Input: dimensioned drawing with shaded views. Units: mm. Origin: part minimum x, y, z. A direction names the side the tool comes from. Give positions to 0.01 mm unless a question says otherwise; leave off trailing zeros. Order: outer loops, then holes, each group sorted by start corner. A loop starts at its lowest first (then second) coordinate and runs counter-clockwise, first axis right, second up. Notation, with made-up numbers: M 73.5,12 L 114.5,12 A18 cw 114.5,32 Z; hole C 34,-23 d8. An arc over 180 degrees is marked long. Answer in a Markdown table with one row per item. Add a question column.
(1) Section query C-C, the plane z = 1.75. Return loops of the section in (x, y), plus the area to 3 significant figures.
(2) Section query A-A, the plane x = 8. Return loops of the section in (y, z).
(3) Material intervals for line 1 along Y through (x, z) = (8, 3.5); line 2 along Z through (x, y) = (2.25, 5.75); line 3 along X through (y, z) = (9.25, 5.75), sorted ascending.
(4) Mould query, pull axis Y, two halves, no side actions, for the marked faces 3, 4 and 5. Classes: pulls with the +Y half, pulls with the -Y half, needs draft (parallel to the pull), parting line crosses it, or undercut.
(5) Section query D-D, the plane z = 7.75. Return loops of the section in (x, y), plus the area to 3 significant figures.
(6) Set-up query: the marked faces 1 and 2. Return all of +Z, -Z, +X, -X, +Y, -Y with unobstructed straight access to the full face (end or side cutting, diameter ignored); none if empty.
(7) Pin query (flat end, axial travel): P1, Ø1.5, axis at x = 10.5, z = 2.5, coming from the +Y side; P2, Ø2, axis at y = 10.5, z = 2.5, coming from the -X side; P3, Ø2, axis at y = 9, z = 3.5, coming from the -X side. Return the tip coordinate at first contact, or that it passes through.
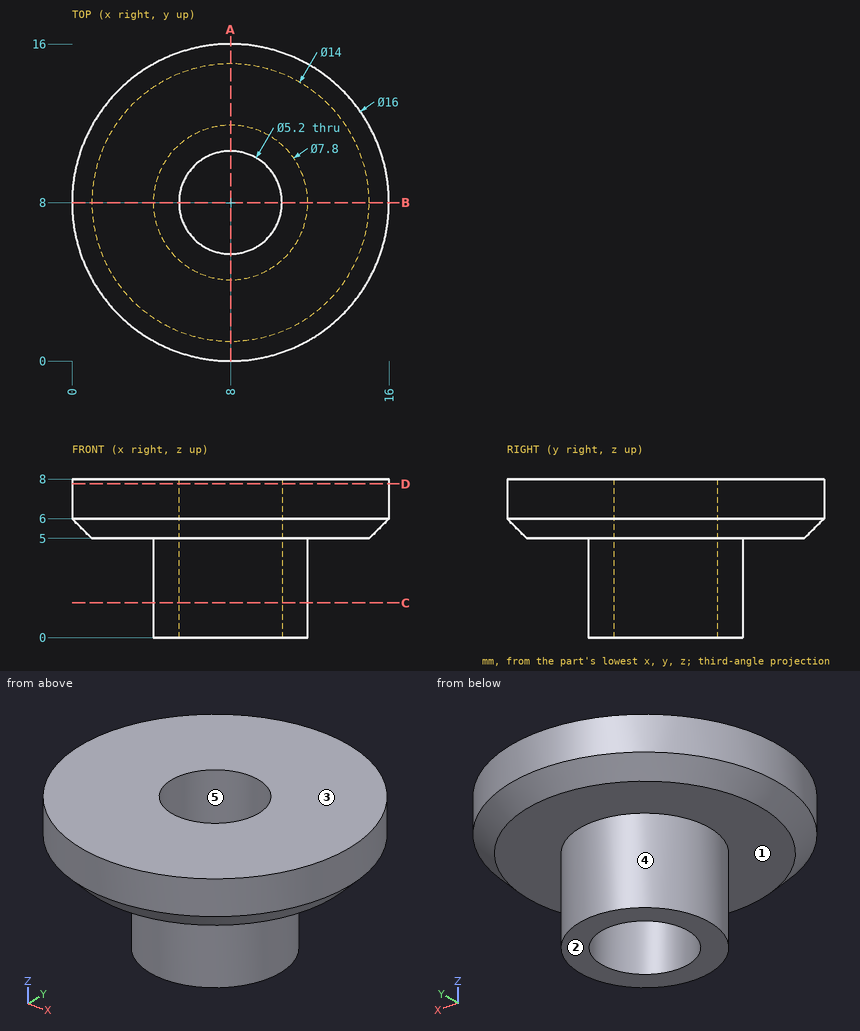
Values follow:
| question | item | result |
|---|---|---|
| 1 | outline | C 8,8 d7.8; hole C 8,8 d5.2 |
| 1 | area | 26.5 mm² |
| 2 | outline | M 0,6 L 1,5 L 4.1,5 L 4.1,0 L 5.4,0 L 5.4,8 L 0,8 Z; M 10.6,0 L 11.9,0 L 11.9,5 L 15,5 L 16,6 L 16,8 L 10.6,8 Z |
| 3 | line 1 | y = 4.1 to 5.4, 10.6 to 11.9 |
| 3 | line 2 | z = 5 to 8 |
| 3 | line 3 | x = 0.35 to 5.72, 10.28 to 15.65 |
| 4 | face 3 | needs draft |
| 4 | face 4 | parting line crosses it |
| 4 | face 5 | undercut |
| 5 | outline | C 8,8 d16; hole C 8,8 d5.2 |
| 5 | area | 180 mm² |
| 6 | face 1 | -Z |
| 6 | face 2 | -Z, +X, -X, +Y, -Y |
| 7 | P1 | stops at y = 11.49 |
| 7 | P2 | stops at x = 4.4 |
| 7 | P3 | stops at x = 4.1 |
